```python
from build123d import *

# Parameters (mm, degrees)
ESQUISSE2_R                  = 3
ENL_V_MAT_EXTRU_1_DEPTH      = 10
ENL_V_MAT_EXTRU_1_DEPTH_BACK = 448


with BuildPart() as part:
    # Esquisse1 → Révolution1 (revolve)
    with BuildSketch(Plane.XY, mode=Mode.PRIVATE) as r_volution1_sk:
        with BuildLine():
            Line((-18.039330687, 17.767949192), (75.138971442, 42.735))
            Line((75.138971442, 42.735), (105.960669313, 50.993649054))
            Line((105.960669313, 50.993649054), (105.960669313, 54.493649054))
            Line((105.960669313, 54.493649054), (1.640278983, 26.81375317))
            Line((1.640278983, 26.81375317), (-16.359721017, 26.81375317))
            Line((-16.359721017, 26.81375317), (-19.950707197, 33.033523683))
            Line((-19.950707197, 33.033523683), (-30.864182635, 51.93621763))
            Line((-30.864182635, 51.93621763), (-32.699704078, 55.033523683))
            Line((-32.699704078, 55.033523683), (-32.699704078, 58.335972539))
            Line((-32.699704078, 58.335972539), (-32.699704078, 59.3))
            Line((-32.699704078, 59.3), (-32.699704078, 77.3))
            Line((-32.699704078, 77.3), (-42.699704078, 77.3))
            Line((-42.699704078, 77.3), (-42.699704078, 59.3))
            Line((-42.699704078, 59.3), (-68.850994622, 59.3))
            Line((-68.850994622, 59.3), (-68.850994622, 55))
            Line((-68.850994622, 55), (-75.850994622, 55))
            Line((-75.850994622, 55), (-75.850994622, 59.3))
            Line((-75.850994622, 59.3), (-80.850994622, 59.3))
            Line((-80.850994622, 59.3), (-80.850994622, 55))
            Line((-80.850994622, 55), (-87.850994622, 55))
            Line((-87.850994622, 55), (-87.850994622, 59.3))
            Line((-87.850994622, 59.3), (-92.850994622, 59.3))
            Line((-92.850994622, 59.3), (-92.850994622, 55))
            Line((-92.850994622, 55), (-99.850994622, 55))
            Line((-99.850994622, 55), (-99.850994622, 59.3))
            Line((-99.850994622, 59.3), (-104.850994622, 59.3))
            Line((-104.850994622, 59.3), (-99.850994622, 50))
            Line((-99.850994622, 50), (-49.762698238, 50))
            Line((-49.762698238, 50), (-39.852583688, 50))
            ThreePointArc((-39.852583688, 50), (-38.255739202, 49.559662211), (-36.97118184, 48.513850534))
            Line((-36.97118184, 48.513850534), (-19.283196137, 17.877360613))
            ThreePointArc((-19.283196137, 17.877360613), (-18.675390795, 17.662044942), (-18.039330687, 17.767949192))
        make_face()
    revolve(r_volution1_sk.sketch.rotate(Axis((-113.603789782, 0, 0), (1, 0, 0)), 90), axis=Axis((-113.603789782, 0, 0), (1, 0, 0)))  # turned: the seam where the file's is

    # Esquisse2 → Enlèv. mat.-Extru.1 (cut, two sides)
    with BuildSketch(Plane(origin=(0, 0, 0), x_dir=(0, 0, -1), z_dir=(1, 0, 0))) as enl_v_mat_extru_1_sk:
        with Locations(Location((-69.726916044, 13.905652772, 0), (0, 0, 180))):  # turned: the seam where the file's is
            Circle(ESQUISSE2_R)
        with Locations(Location((-46.906106579, -53.432454235, 0), (0, 0, 180))):  # turned: the seam where the file's is
            Circle(ESQUISSE2_R)
        with Locations(Location((22.820809465, -67.338107008, 0), (0, 0, 180))):  # turned: the seam where the file's is
            Circle(ESQUISSE2_R)
        with Locations(Location((69.726916044, -13.905652772, 0), (0, 0, 180))):  # turned: the seam where the file's is
            Circle(ESQUISSE2_R)
        with Locations(Location((46.906106579, 53.432454235, 0), (0, 0, 180))):  # turned: the seam where the file's is
            Circle(ESQUISSE2_R)
        with Locations(Location((-22.820809465, 67.338107008, 0), (0, 0, 180))):  # turned: the seam where the file's is
            Circle(ESQUISSE2_R)
    extrude(amount=ENL_V_MAT_EXTRU_1_DEPTH, mode=Mode.SUBTRACT)
    extrude(enl_v_mat_extru_1_sk.sketch, amount=-ENL_V_MAT_EXTRU_1_DEPTH_BACK, mode=Mode.SUBTRACT)


solid = part.part
```
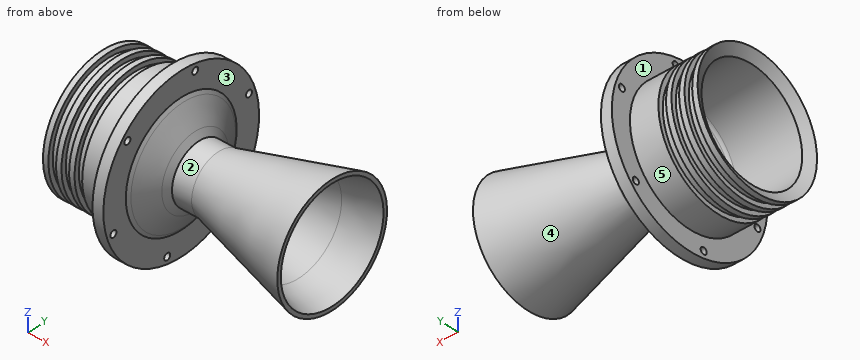
Verification items for the finished model (mm, model axes). Face numbers are marked on the shaded views. A direction names the side the tool comes from. Coordinates: 2 decimals unless noted, no trailing zeros. Order: outer loops, then holes, each group sorted by start corner. A loop starts at its lowest first (then second) coordinate and runs counter-clockwise, first axis right, second up. Notation, with made-up numbers: (55, 72) -> (68, 72) arc R9 ccw to (68, 79) -> close; hole circle Ø7 at (1, 49.5). An arc over 180 degrees is marked (long way). Answer as CSV lines item,"result". Start each with the question number.
1) Release check for a two-part mould opening along X. For the marked faces 3, 4 and 5 record: released by +X, released by -X, zero draft, split by the parting line, or undercut.
2) Cross-section at A-A, the plane x = 16. Record the boundary of the cut face in (y, z).
3) Set-up check for the marked faces 1 and 2: record each of +Z, -Z, +X, -X, +Y, -Y from which the full face is reachable in a straight line by a thin tool's end or side.
4) Gauge pin test, flat ends, axial feed: pin 1 Ø9.5 at (y, z) = (53.43, -46.91) entering from -X; pin 2 Ø8 at (x, y) = (-31, 19) entering from -Z; pin 3 Ø1 at (y, z) = (-4, -57) entering from -X. Record the tip position at first contact, or that the pin passes through.
5) Cross-section at B-B, the plane x = -13.5. Record the boundary of the cut face in (y, z), then the cut area to 3 significant figures.
6) Material ranges on L1, parallel to Z at x = -59.5, y = 2; L2, parallel to X at y = 63, z = 29; L3, parallel to Z at x = -21, y = 12, recorded low to high. Write a range as [from, to].
Conclusion:
1,face 3,"released by +X"
1,face 4,"undercut"
1,face 5,"zero draft"
2,outline,"circle Ø61.25 at (0, 0); hole circle Ø53.78 at (0, 0)"
3,face 1,"-X"
3,face 2,"none"
4,pin 1,"stops at x = -42.7"
4,pin 2,"stops at z = -75.75"
4,pin 3,"stops at x = -103.96"
5,outline,"circle Ø53.63 at (0, 0); hole circle Ø37.97 at (0, 0)"
5,area,"1,130 mm²"
6,L1,"z = [-59.27, -49.96], [49.96, 59.27]"
6,L2,"x = [-42.7, -32.7]"
6,L3,"z = [-32.72, -17.05], [17.05, 32.72]"
